from build123d import *

# Parameters (mm, degrees)
EXTRUDE1_DEPTH        = 102
SKETCH3_W             = 38
SKETCH3_H             = 40
EXTRUDE3_DEPTH        = 54
SKETCH4_R             = 10
EXTRUDE4_DEPTH        = 127.585939188
M6_TAPPED_HOLE1_D     = 5
M6_TAPPED_HOLE1_DEPTH = 14
M6_TAPPED_HOLE1_TIP   = 1.502151548
M6_TAPPED_HOLE2_D     = 5
M6_TAPPED_HOLE2_DEPTH = 10
M6_TAPPED_HOLE2_TIP   = 1.502151548


with BuildPart() as part:
    # Sketch1 → Extrude1 (new body)
    with BuildSketch(Plane(origin=(0, 0, 0), x_dir=(0, 0, -1), z_dir=(1, 0, 0))):
        with BuildLine():
            Line((-5.361015491, 52), (-5.361015491, 28))
            Line((-5.361015491, 28), (-8.361015491, 28))
            Line((-8.361015491, 28), (-8.361015491, 25))
            Line((-8.361015491, 25), (45.638984509, 25))
            Line((45.638984509, 25), (45.638984509, 40))
            ThreePointArc((45.638984509, 40), (42.124265884, 48.485281374), (33.638984509, 52))
            Line((33.638984509, 52), (-5.361015491, 52))
        make_face()
    extrude(amount=EXTRUDE1_DEPTH)

    # Sketch3 → Extrude3 (add)
    with BuildSketch(Plane.XY.offset(8.361015491)):
        with Locations((51, 5)):
            Rectangle(SKETCH3_W, SKETCH3_H)
    extrude(amount=-EXTRUDE3_DEPTH)

    # Sketch4 → Extrude4 (cut, through all)
    with BuildSketch(Plane.XY.offset(8.361015491)):
        with Locations((51, 0)):
            Circle(SKETCH4_R)
    extrude(amount=-EXTRUDE4_DEPTH, mode=Mode.SUBTRACT)

    # M6 Tapped Hole1
    with Locations(Plane(origin=(22, 40, 5.361015491), x_dir=(1, 0, 0), z_dir=(0, 0, 1))):
        with Locations((0, 0), (58, 0)):
            Hole(M6_TAPPED_HOLE1_D / 2, depth=M6_TAPPED_HOLE1_DEPTH)
            with Locations((0, 0, -(M6_TAPPED_HOLE1_DEPTH + M6_TAPPED_HOLE1_TIP / 2))):  # 118° drill point
                Cone(0, M6_TAPPED_HOLE1_D / 2, M6_TAPPED_HOLE1_TIP, mode=Mode.SUBTRACT)

    # M6 Tapped Hole2
    with Locations(Plane(origin=(39, -15, -18.638984509), x_dir=(-1, 0, 0), z_dir=(0, -1, 0))):
        with Locations((0, 0), (-24, 0)):
            Hole(M6_TAPPED_HOLE2_D / 2, depth=M6_TAPPED_HOLE2_DEPTH)
            with Locations((0, 0, -(M6_TAPPED_HOLE2_DEPTH + M6_TAPPED_HOLE2_TIP / 2))):  # 118° drill point
                Cone(0, M6_TAPPED_HOLE2_D / 2, M6_TAPPED_HOLE2_TIP, mode=Mode.SUBTRACT)


solid = part.part
Model file for the job. Use its own axes, mm. A direction names the side the tool comes from. Give positions to 0.01 mm unless a question says otherwise; leave off trailing zeros. Order: outer loops, then holes, each group sorted by start corner. A loop starts at its lowest first (then second) coordinate and runs counter-clockwise, first axis right, second up. Notation, with made-up numbers: (30.25, 60) - (56.25, 60) arc R23 ccw to (56.25, 69) - close; hole circle Ø2 at (26.25, 74.25). An arc over 180 degrees is marked (long way). Return JSON: item names as keys, results as strings.
1) Cut at B-B, the plane y = 8. Give the cut face in (x, z).
Geometry says:
{"outline": "(32, -45.64) - (45, -45.64) - (45, 8.36) - (32, 8.36) - close; (57, -45.64) - (70, -45.64) - (70, 8.36) - (57, 8.36) - close"}
2) Pull direction X, two halves, no side cores. Call faces 6 (the cylindrical face through (50.29, 48.39, -42.22)), 7 (the cylindrical face through (41, 0, -18)), 8 (the flat face through (32, 5, -18)): pulls with the +X half, pulls with the -X half, needs draft (parallel to the pull), parting line crosses it, or undercut.
Geometry says:
{"face 6": "needs draft", "face 7": "undercut", "face 8": "pulls with the -X half"}
3) Cut at C-C, the plane z = -13.5. Give the cut face in (x, y).
Geometry says:
{"outline": "(0, 25) - (32, 25) - (32, -15) - (70, -15) - (70, 25) - (102, 25) - (102, 52) - (0, 52) - close; hole circle Ø20 at (51, 0)"}
4) 3-axis set-ups, long thin cutter, end or side, ignore diameter. For faces 1 (the flat face through (50, 28, 7)), 2 (the cylindrical face through (82, 38.5, -1.7)), 3 (the flat face through (16, 25, -18)), 4 (the flat face through (86, 25, -18)), 5 (the cylindrical face through (41.385, -9.93, -19.39)): which of +Z, -Z, +X, -X, +Y, -Y reach the whole face in a straight line?
Geometry says:
{"face 1": "+Z, +X, -X, +Y", "face 2": "+Z", "face 3": "+Z, -Z, -X, -Y", "face 4": "+Z, -Z, +X, -Y", "face 5": "-Y"}
5) Cut at D-D, the plane x = 87. Give the cut face in (y, z), plus the area to 3 significant figures.
Geometry says:
{"outline": "(25, -45.64) - (40, -45.64) arc R12 ccw to (52, -33.64) - (52, 5.36) - (28, 5.36) - (28, 8.36) - (25, 8.36) - close", "area": "1,360 mm²"}
6) Cut at A-A, the plane x = 51. Give the cut face in (y, z).
Geometry says:
{"outline": "(-15, -45.64) - (-10, -45.64) - (-10, 8.36) - (-15, 8.36) - close; (10, -45.64) - (40, -45.64) arc R12 ccw to (52, -33.64) - (52, 5.36) - (28, 5.36) - (28, 8.36) - (10, 8.36) - close"}
7) Flat gauge pins, fed straight in: P1, Ø1.5, axis at y = 5.5, z = -32, coming from the +X side; P2, Ø9.5, axis at x = 92.5, z = -26.5, coming from the -Y side; P3, Ø1.5, axis at x = 44.5, z = 7, coming from the +Y side. Where does each tip first touch, or does it go through?
Geometry says:
{"P1": "x = 70", "P2": "y = 25", "P3": "y = 28"}
8) Probe line 1 (X direction, y = 40, z = -2.75); line 2 (Y direction, x = 80, z = 0); line 3 (Z direction, x = 63, y = -7.25). List the from-to ranges inside material, lowest first. Write a range as from..to.
Geometry says:
{"line 1": "0..19.5, 24.5..77.5, 82.5..102", "line 2": "25..37.5, 42.5..52", "line 3": "-45.64..-21.14, -16.14..8.36"}
